Build history of the part. All positions in model axes, mm. Face numbers are marked on the shaded views. A direction names the side the tool comes from. Round coordinates to 2 decimals unless told otherwise and drop trailing zeros. Loops run counter-clockwise (first coordinate to the right, second up) from the corner with the lowest first, then second, coordinate; pieces in that order, holes last. Notation, with made-up numbers: (-8.5, -22) -> (23.5, -22) arc R24 ccw to (23.5, 13) -> close; hole circle Ø7 at (21, -23.5). An arc over 180 degrees is marked (long way). Put each result on its own line as item: value. Start each with the question number.
Item 1: Cut at A-A, the plane y = 19.5. List the corners of the cut face in (x, z), plus the area to 3 significant figures.
Item 2: Drill centre lines: probe 1 along Z at (x, y) = (0, 36.5); probe 2 along X at (y, z) = (72, -0.5). Where is each one in solid material? Low to high. Write a range as [from, to].
Item 3: Cut at B-B, the plane y = 63.5. List the corners of the cut face in (x, z).
Item 4: Flat gauge pins, fed straight in: pin 1 Ø1.7 at (x, z) = (1, -0.5) entering from -Y; pin 2 Ø0.8 at (x, y) = (2.5, 3) entering from +Z; pin 3 Ø5 at (y, z) = (50, -1) entering from -X. Where does each tip first touch, or does it go through?
Item 5: Tool access for the marked faces 1 and 2: list every direction of +Z, -Z, +X, -X, +Y, -Y with a clear straight run to the whole face (end or side of a thin tool).
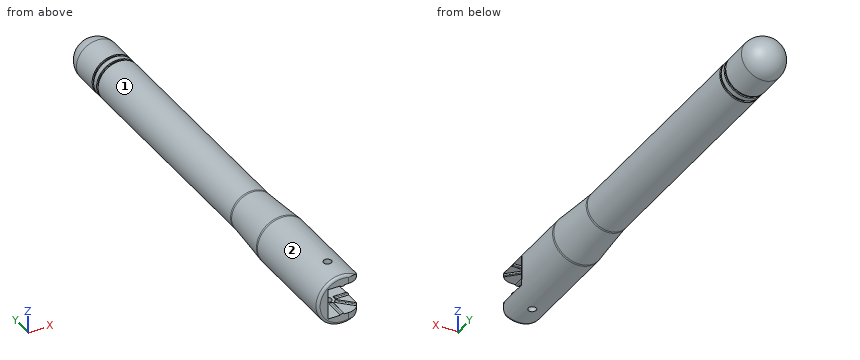
```python
from build123d import *

# Parameters (mm, degrees)
ESQUISSE3_W                  = 7.5
ESQUISSE3_H                  = 5.8
ENL_V_MAT_EXTRU_1_DEPTH      = 8
CONG_1_R                     = 0.5
ENL_V_MAT_EXTRU_2_DEPTH      = 87.712791632
ENL_V_MAT_EXTRU_2_DEPTH_BACK = 87.712791632
ESQUISSE4_R                  = 0.75
ESQUISSE5_W                  = 0.75
ESQUISSE5_H                  = 3.75
ESQUISSE5_W_2                = 2.511980861
ESQUISSE5_H_2                = 0.75
BOSS_EXTRU_1_DEPTH           = 0.2
CONG_2_R                     = 0.2
CONG_2_OF_SYM_TRIE1_R        = 0.2
ENL_V_MAT_EXTRU_3_DEPTH      = 87.919895497


with BuildPart() as part:
    # Esquisse2 → Révolution1 (revolve)
    with BuildSketch(Plane.XY):
        with BuildLine():
            Line((4.014003451, 30.213287326), (4.735996549, 20.586712674))
            ThreePointArc((4.735996549, 20.586712674), (4.746497911, 20.399868856), (4.75, 20.212762933))
            Line((4.75, 20.212762933), (4.75, 0))
            Line((4.75, 0), (1, 0))
            Line((1, 0), (1, 82.452202))
            Line((1, 82.452202), (0, 82.452202))
            Line((0, 82.452202), (0, 86.452202))
            ThreePointArc((0, 86.452202), (2.828427125, 85.280629125), (4, 82.452202))
            Line((4, 82.452202), (4, 77.152202))
            Line((4, 77.152202), (3.75, 77.152202))
            Line((3.75, 77.152202), (3.75, 76.652202))
            Line((3.75, 76.652202), (4, 76.652202))
            Line((4, 76.652202), (4, 75.652202))
            Line((4, 75.652202), (3.75, 75.652202))
            Line((3.75, 75.652202), (3.75, 75.152202))
            Line((3.75, 75.152202), (4, 75.152202))
            Line((4, 75.152202), (4, 30.587237067))
            ThreePointArc((4, 30.587237067), (4.003502089, 30.400131144), (4.014003451, 30.213287326))
        make_face()
    revolve(axis=Axis((0, 0, 0), (0, 1, 0)))

    # Esquisse3 → Enlèv. mat.-Extru.1 (cut)
    with BuildSketch(Plane.XZ):
        with Locations((1, 0)):
            Rectangle(ESQUISSE3_W, ESQUISSE3_H)
    extrude(amount=-ENL_V_MAT_EXTRU_1_DEPTH, mode=Mode.SUBTRACT)

    # Congé1
    cong_1_edges = [part.edges().sort_by_distance(p)[0] for p in [
        (-4.75, 0, 0),
    ]]
    fillet(cong_1_edges, radius=CONG_1_R)

    # Esquisse4 → Enlèv. mat.-Extru.2 (cut, two sides: drawn at the far end of the back side and taken through both)
    with BuildSketch(Plane.XY.offset(-ENL_V_MAT_EXTRU_2_DEPTH_BACK)):
        with Locations((0, 5)):
            Circle(ESQUISSE4_R)
        with BuildLine():
            Line((1.161980861, 0), (3.761980861, 0))
            Line((3.761980861, 0), (3.761980861, 2.6))
            ThreePointArc((3.761980861, 2.6), (3.000458492, 0.761522369), (1.161980861, 0))
        make_face()
        Polygon((3.761980861, 8), (4.75, 10), (4.75, 8), align=None)
    extrude(amount=ENL_V_MAT_EXTRU_2_DEPTH + ENL_V_MAT_EXTRU_2_DEPTH_BACK, mode=Mode.SUBTRACT)

    # Esquisse5 → Boss.-Extru.1 (add)
    with BuildSketch(Plane.XY.offset(-2.9)):
        with Locations((0, 1.875)):
            Rectangle(ESQUISSE5_W, ESQUISSE5_H)
        Polygon((0.618718434, 3.850951481), (1.149048519, 4.381281566), (4.027145904, 1.503184182), (3.496815818, 0.972854096), align=None)
        with Locations((2.50599043, 5)):
            Rectangle(ESQUISSE5_W_2, ESQUISSE5_H_2)
    boss_extru_1 = extrude(amount=BOSS_EXTRU_1_DEPTH)

    # Congé2
    cong_2_edges = [part.edges().sort_by_distance(p)[0] for p in [
        (2.505990431, 5.375, -2.7),
        (2.505990431, 4.625, -2.7),
        (2.588097212, 2.942232874, -2.7),
        (2.057767126, 2.411902788, -2.7),
        (-0.375, 1.875, -2.7),
        (0.375, 1.875, -2.7),
    ]]
    fillet(cong_2_edges, radius=CONG_2_R - 0.0001)  # a hair under: the kernel refuses the full size

    # Symétrie1: Boss.-Extru.1 across plane
    add(boss_extru_1.mirror(Plane.XY))

    # Congé2 of Symétrie1
    cong_2_of_sym_trie1_edges = [part.edges().sort_by_distance(p)[0] for p in [
        (2.505990431, 5.375, 2.7),
        (2.505990431, 4.625, 2.7),
        (2.588097212, 2.942232874, 2.7),
        (2.057767126, 2.411902788, 2.7),
        (-0.375, 1.875, 2.7),
        (0.375, 1.875, 2.7),
    ]]
    fillet(cong_2_of_sym_trie1_edges, radius=CONG_2_OF_SYM_TRIE1_R - 0.0001)  # a hair under: the kernel refuses the full size

    # Esquisse6 → Enlèv. mat.-Extru.3 (cut, through all)
    with BuildSketch(Plane.XY.offset(2.9)):
        with BuildLine():
            Line((4.027145904, 1.503184182), (3.658059706, 1.87227038))
            ThreePointArc((3.658059706, 1.87227038), (3.516870908, 1.49795968), (3.319930166, 1.149739748))
            Line((3.319930166, 1.149739748), (3.496815818, 0.972854096))
            Line((3.496815818, 0.972854096), (4.027145904, 1.503184182))
        make_face()
    extrude(amount=-ENL_V_MAT_EXTRU_3_DEPTH, mode=Mode.SUBTRACT)


solid = part.part
```
Reply:
1. outline: circle Ø9.5 at (0, 0); hole circle Ø2 at (0, 0)
1. area: 67.7 mm^2
2. probe 1: z = [-4, -1], [1, 4]
2. probe 2: x = [-3.97, -0.87], [0.87, 3.97]
3. outline: circle Ø8 at (0, 0); hole circle Ø2 at (0, 0)
4. pin 1: stops at y = 8
4. pin 2: stops at z = 4.26
4. pin 3: stops at x = -4
5. face 1: +Y
5. face 2: +Y, -Y
